Verification items for the finished model (mm, model axes). A direction names the side the tool comes from. Round coordinates to 2 decimals unless told otherwise and drop trailing zeros. Write each loop counter-clockwise with the first axis right and the second up, starting at its lowest first coordinate (ties: lowest second). Pieces come first, ordered by that corner, then holes. Notation, with made-up numbers: M 85,-26.5 L 123,-26.5 A16 ccw 123,-16.5 Z; hole C 33.5,36 d7. An arc over 180 degrees is marked long. Write each question's results on one line, items separated by ' | '.
from build123d import *

# Parameters (mm, degrees)
BOSS_EXTRUDE1_DEPTH                  = 62.5
BOSS_EXTRUDE2_REACH                  = 289.283
SKETCH6_W                            = 14
SKETCH6_H                            = 267.143428259
CUT_EXTRUDE1_DEPTH                   = 10
RIB1_REACH                           = 288.004
SKETCH7_WALL_W                       = 627.230719128
SKETCH7_WALL_H                       = 15
FILLET1_R                            = 20
CUT_EXTRUDE2_DEPTH                   = 30
F_20_0_20_DIAMETER_HOLE1_D           = 20
F_20_0_20_DIAMETER_HOLE1_CSINK_D     = 20.05
F_20_0_20_DIAMETER_HOLE1_CSINK_ANGLE = 90
F_20_0_20_DIAMETER_HOLE2_D           = 20
F_20_0_20_DIAMETER_HOLE2_DEPTH       = 40
F_20_0_20_DIAMETER_HOLE2_CSINK_D     = 20.05
F_20_0_20_DIAMETER_HOLE2_CSINK_ANGLE = 90
F_20_0_20_DIAMETER_HOLE2_TIP         = 6.00860619


with BuildPart() as part:
    # Sketch1 → Boss-Extrude1 (new, symmetric)
    with BuildSketch(Plane(origin=(0, 0, 0), x_dir=(0, 0, -1), z_dir=(1, 0, 0))):
        Polygon((0, 0), (0, 90), (190, 90), (190, 150), (215, 150), (215, 65), (25, 65), (25, 0), align=None)
    extrude(amount=BOSS_EXTRUDE1_DEPTH, both=True)

    # Boss-Extrude2: up to this face of the body (flat: up to its plane)
    boss_extrude2_end = Plane(part.part.faces().sort_by_distance((0, 90, -95))[0])
    # Sketch2 → Boss-Extrude2 (add, up to the picked face)
    with BuildSketch(Plane(origin=(0, 45, 45), x_dir=(1, 0, 0), z_dir=(0, 0.7071067811865464, 0.7071067811865488)), mode=Mode.PRIVATE) as boss_extrude2_sk1:
        with BuildLine():
            Line((-40, 63.639610307), (-40, 148.639610307))
            ThreePointArc((-40, 148.639610307), (0, 188.639610307), (40, 148.639610307))
            Line((40, 148.639610307), (40, 63.639610307))
            Line((40, 63.639610307), (-40, 63.639610307))
        make_face()
    boss_extrude2_tool1 = split(extrude(boss_extrude2_sk1.sketch, amount=-BOSS_EXTRUDE2_REACH, mode=Mode.PRIVATE), bisect_by=boss_extrude2_end, keep=Keep.BOTH, mode=Mode.PRIVATE)
    add(boss_extrude2_tool1.solids().sort_by(Axis((0, 131.401312, -41.401312), (0, -0.7071067811865464, -0.7071067811865488)))[0])

    # Sketch5 → CBORE for M24 Hex Head Bolt1 (revolve, cut)
    with BuildSketch(Plane(origin=(0, 150.104076401, -60.104076401), x_dir=(0, -0.7071067811865487, 0.7071067811865465), z_dir=(1, 0, 0))):
        Polygon((0, 0), (0, 215.667568262), (13, 215.667568262), (13, 15), (22.2845, 15), (22.2845, 0.025), (22.3095, 0), align=None)
    revolve(axis=Axis((0, 154.594204461, -55.61394834), (0, -0.7071067811865465, -0.7071067811865486)), mode=Mode.SUBTRACT)

    # Sketch6 → Cut-Extrude1 (cut)
    with BuildSketch(Plane(origin=(0, 45, 45), x_dir=(1, 0, 0), z_dir=(0, 0.7071067811865465, 0.7071067811865487))):
        with Locations((0, 148.639610307)):
            Rectangle(SKETCH6_W, SKETCH6_H)
    extrude(amount=-CUT_EXTRUDE1_DEPTH, mode=Mode.SUBTRACT)

    # Sketch7 wall → Rib1 (add, up to next)
    with BuildSketch(Plane(origin=(0, 130, -163.388347649), x_dir=(0, 0, -1), z_dir=(0, 1, 0)), mode=Mode.PRIVATE) as rib1_sk1:
        Rectangle(SKETCH7_WALL_W, SKETCH7_WALL_H)
    rib1_tool1 = extrude(rib1_sk1.sketch, amount=-RIB1_REACH, mode=Mode.PRIVATE) - part.part
    add(rib1_tool1.solids().sort_by_distance((0, 130, -163.388347649))[0])

    # Fillet1
    fillet1_edges = [part.edges().sort_by_distance(p)[0] for p in [
        (62.5, 0, -12.5),
        (-62.5, 150, -202.5),
        (-62.5, 0, -12.5),
        (62.5, 150, -202.5),
    ]]
    fillet(fillet1_edges, radius=FILLET1_R)

    # Sketch8 → Cut-Extrude2 (cut)
    with BuildSketch(Plane(origin=(0, 90, 0), x_dir=(1, 0, 0), z_dir=(0, 1, 0))):
        with BuildLine():
            Line((77.5, 150), (77.5, 50))
            ThreePointArc((77.5, 50), (62.5, 35), (47.5, 50))
            Line((47.5, 50), (47.5, 150))
            ThreePointArc((47.5, 150), (62.5, 165), (77.5, 150))
        make_face()
        with BuildLine():
            Line((-77.5, 150), (-77.5, 50))
            ThreePointArc((-77.5, 50), (-62.5, 35), (-47.5, 50))
            Line((-47.5, 50), (-47.5, 150))
            ThreePointArc((-47.5, 150), (-62.5, 165), (-77.5, 150))
        make_face()
    extrude(amount=-CUT_EXTRUDE2_DEPTH, mode=Mode.SUBTRACT)

    # Ø20.0 (20) Diameter Hole1 (through all)
    with Locations(Plane.XY):
        with Locations((42.5, 20), (-42.5, 20)):
            CounterSinkHole(F_20_0_20_DIAMETER_HOLE1_D / 2, F_20_0_20_DIAMETER_HOLE1_CSINK_D / 2, counter_sink_angle=F_20_0_20_DIAMETER_HOLE1_CSINK_ANGLE)

    # Ø20.0 (20) Diameter Hole2
    with Locations(Plane(origin=(0, 0, -215), x_dir=(-1, 0, 0), z_dir=(0, 0, -1))):
        with Locations((-42.5, 130), (42.5, 130)):
            CounterSinkHole(F_20_0_20_DIAMETER_HOLE2_D / 2, F_20_0_20_DIAMETER_HOLE2_CSINK_D / 2, depth=F_20_0_20_DIAMETER_HOLE2_DEPTH, counter_sink_angle=F_20_0_20_DIAMETER_HOLE2_CSINK_ANGLE)
            with Locations((0, 0, -(F_20_0_20_DIAMETER_HOLE2_DEPTH + F_20_0_20_DIAMETER_HOLE2_TIP / 2))):  # 118° drill point
                Cone(0, F_20_0_20_DIAMETER_HOLE2_D / 2, F_20_0_20_DIAMETER_HOLE2_TIP, mode=Mode.SUBTRACT)


solid = part.part
1) Draft check along Y on faces 6 (the flat face through (7, 105, -22)), 7 (the flat face through (9.592, 146.28, -77.493)), 8 (the flat face through (1, 150, -202)). Enter one of: pulls with the +Y half, pulls with the -Y half, needs draft (parallel to the pull), parting line crosses it, or undercut.
Calculated:
face 6: needs draft | face 7: undercut | face 8: pulls with the +Y half
2) Sectioned sample at D-D, the plane x = 50. Count the separate pieces of the cut face and the enclosed holes in it, and give its area (3 significant figures).
Calculated:
separate pieces: 4 | enclosed holes: 0 | area: 4,850 mm²
3) Sectioned sample at B-B, the plane x = 4.5. Record the cut outline in (y, z).
Calculated:
outline: M 0,-25 L 65,-25 L 65,-127.96 L 130.87,-62.09 L 124.06,-55.28 L 127.6,-51.74 L 75.86,0 L 0,0 Z; M 65,-215 L 150,-215 L 150,-190 L 130,-190 L 130,-136.42 L 171.14,-95.28 L 158.47,-82.61 L 154.93,-86.14 L 148.12,-79.33 L 65,-162.46 Z
4) Access from +Z, -Z, +X, -X, +Y, -Y to the whole of each face (thin tool, end or side, straight path). Record for faces 1 (the cylindrical face through (-49.87, 136.76, -202.31)), 2 (the cylindrical face through (52.01, 77.68, -39.28)), 3 (the cylindrical face through (-51.78, 77.68, -160.49)), 4 (the flat face through (1, 65, -121)), 5 (the flat face through (43, 90, -116)).
Calculated:
face 1: -Z | face 2: +X, +Y, -Y | face 3: -X, +Y, -Y | face 4: -Z, +X, -X, -Y | face 5: +X, +Y
5) Sectioned sample at A-A, the plane z = -182.5. Record the cut outline in (x, y), and give its area (4 significant figures).
Calculated:
outline: M -62.5,65 L 62.5,65 L 62.5,90 L 7.5,90 L 7.5,130 L -7.5,130 L -7.5,90 L -62.5,90 Z | area: 3,725 mm²
6) Material ranges on line 1 (X direction, y = 20, z = -13); line 2 (Y direction, x = -42.5, z = -201); line 3 (Y direction, x = 42.5, z = -5.75), recorded low to high. Write a range as [from, to].
Calculated:
line 1: x = [-62.5, -52.5], [-32.5, 32.5], [52.5, 62.5] | line 2: y = [65, 120], [140, 150] | line 3: y = [0, 10], [30, 90]
7) Depth check by flat-ended pin: P1, Ø15.5, axis at y = 91.5, z = -14, coming from the -X side; P2, Ø12, axis at x = -42.5, y = 20, coming from the +Z side; P3, Ø16, axis at x = 42.5, y = 130, coming from the +Z side; P4, Ø20, axis at y = 83.5, z = -99.5, coming from the +X side. Enter the tip coordinate at first touch or a pass-through.
Calculated:
P1: stops at x = -62.5 | P2: passes through | P3: stops at z = -32.4 | P4: stops at x = 47.5
8) Sectioned sample at C-C, the plane y = 50. Record the cut outline in (x, z).
Calculated:
outline: M -62.5,-25 L 62.5,-25 L 62.5,0 L -62.5,0 Z
